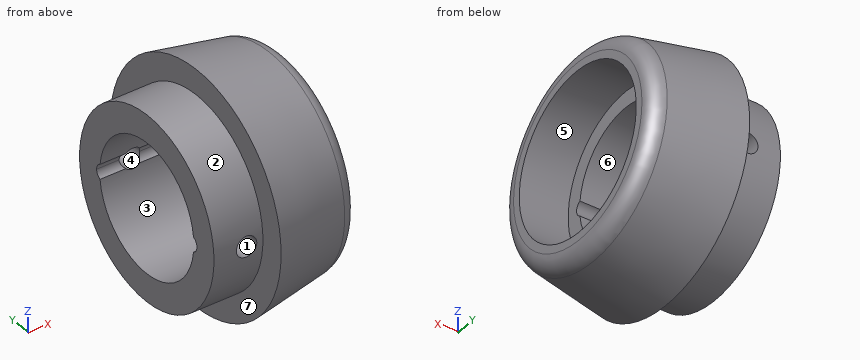
```python
from build123d import *

# Parameters (mm, degrees)
F2_R          = 2.54
F4_DEPTH      = 21.083
F5_R          = 1.5875
F6_DEPTH      = 18.162
F6_DEPTH_BACK = 18.162


with BuildPart() as f1:
    # F0 (on Front) → F1 (revolve)
    with BuildSketch(Plane.XZ):
        Polygon((7.62, 18.161), (7.62, 14.2875), (0, 14.2875), (0, 10.0076), (13.462, 10.0076), (13.462, 12.446), (21.082, 12.446), (21.082, 15.7872861857), align=None)
    revolve(axis=Axis((10.541, 0, 0), (1, 0, 0)))

    # F2
    f2_edges = [f1.edges().sort_by_distance(p)[0] for p in [
        (21.082, 0, -15.787286),
    ]]
    fillet(f2_edges, radius=F2_R)

    # F3 (on Right) → F4 (cut, through all)
    with BuildSketch(Plane.YZ):
        with BuildLine():
            ThreePointArc((-9.94156, -1.1477989922), (-10.0076, 0), (-9.94156, 1.1477989922))
            ThreePointArc((-9.94156, 1.1477989922), (-10.668, 0), (-9.94156, -1.1477989922))
        make_face()
        with BuildLine():
            ThreePointArc((9.94156, 1.1477989922), (9.9910763588, 0.574848634), (10.0076, 0))
            ThreePointArc((10.0076, 0), (9.9910763588, -0.574848634), (9.94156, -1.1477989922))
            ThreePointArc((9.94156, -1.1477989922), (10.4711312129, -0.6791828914), (10.668, 0))
            ThreePointArc((10.668, 0), (10.4711312129, 0.6791828914), (9.94156, 1.1477989922))
        make_face()
    extrude(amount=F4_DEPTH, mode=Mode.SUBTRACT)

    # F5 (on Front) → F6 (cut, two sides)
    with BuildSketch(Plane.XZ) as f6_sk:
        with Locations((5.08, 0)):
            Circle(F5_R)
    extrude(amount=-F6_DEPTH, mode=Mode.SUBTRACT)
    extrude(f6_sk.sketch, amount=F6_DEPTH_BACK, mode=Mode.SUBTRACT)


solid = f1.part
```
Here's how the part is built. I have some questions about the finished solid (model axes, mm). Face numbers are marked on the shaded views. A direction names the side the tool comes from. Coordinates: 2 decimals unless noted, no trailing zeros. Order: outer loops, then holes, each group sorted by start corner. A loop starts at its lowest first (then second) coordinate and runs counter-clockwise, first axis right, second up.
Item 1: If we section it at C-C, the plane x = 14.25: List the corners of the cut face in (y, z) for me.
Response values:
outline: circle Ø33.98 at (0, 0); hole circle Ø24.89 at (0, 0)
Item 2: I need wall thicknesses on probe 1 along X at (y, z) = (11.55, 0); probe 2 along Z at (x, y) = (19.75, 11); probe 3 along Y at (x, z) = (9, -2). Which ranges of each line are inside material? Lowest first, please.
Response values:
probe 1: x = 0 to 3.49, 6.67 to 13.46
probe 2: z = -11.47 to -5.82, 5.82 to 11.47
probe 3: y = -17.81 to -9.81, 9.81 to 17.81
Item 3: Which directions (+Z, -Z, +X, -X, +Y, -Y) give clear straight access to the entire face, cutting with the end or side of a thin tool? Please do the marked faces 4, 5, 6 and 7.
Response values:
face 4: +Y, -Y
face 5: +X
face 6: +X, -X
face 7: -X
Item 4: If we section it at B-B, the plane x = 5.08: List the corners of the cut face in (y, z) for me (1 decimal), then the cut area to 3 significant figures.
Response values:
outline: (-14.2, -1.6) arc R14.3 ccw to (14.2, -1.6) - (9.9, -1.6) arc R10 cw to (-9.9, -1.6) - close; (-14.2, 1.6) - (-9.9, 1.6) arc R10 cw to (9.9, 1.6) - (14.2, 1.6) arc R14.3 ccw to start
area: 299 mm2
Item 5: Thinking about a two-plate mould opening in Y: for the marked faces 1, 2 and 3, which applies, pulls with the +Y half, pulls with the -Y half, needs draft (parallel to the pull), parting line crosses it, or undercut?
Response values:
face 1: needs draft
face 2: parting line crosses it
face 3: undercut
Item 6: I'm going to push flat-ended pins straight in: pin 1 Ø1.5 at (x, z) = (9, -7) entering from -Y; pin 2 Ø1.5 at (x, y) = (13, 0.5) entering from -Z; pin 3 Ø1.5 at (x, y) = (18, -11.5) entering from -Z. Where does each tip first touch, or does it pass through?
Response values:
pin 1: stops at y = -16.83
pin 2: stops at z = -17.34
pin 3: stops at z = -12.32
Item 7: If we section it at A-A, the plane y = 0: List the corners of the cut face in (x, z) for me.
Response values:
outline: (0, -14.29) - (7.62, -14.29) - (7.62, -18.16) - (18.98, -16.16) arc R2.54 ccw to (21.08, -13.66) - (21.08, -12.45) - (13.46, -12.45) - (13.46, -10.01) - (0, -10.01) - close; (0, 10.01) - (13.46, 10.01) - (13.46, 12.45) - (21.08, 12.45) - (21.08, 13.66) arc R2.54 ccw to (18.98, 16.16) - (7.62, 18.16) - (7.62, 14.29) - (0, 14.29) - close
